Verification items for the finished model (mm, model axes). Give positions to 0.01 mm unless a question says otherwise; leave off trailing zeros. Write each loop counter-clockwise with the first axis right and the second up, starting at its lowest first coordinate (ties: lowest second). Pieces come first, ordered by that corner, then holes.
from build123d import *

# Parameters (mm, degrees)
F0_W     = 555
F0_H     = 70
F1_DEPTH = 45
F2_R     = 11.85
F3_DEPTH = 45.001
F4_R     = 12
F5_DEPTH = 45.001


with BuildPart() as f1:
    # F0 (on Front) → F1 (new body)
    with BuildSketch(Plane.XZ):
        with Locations((-277.5, -35)):
            Rectangle(F0_W, F0_H)
    extrude(amount=F1_DEPTH)

    # F2 (on face) → F3 (cut, through all)
    with BuildSketch(Plane(origin=(0, 0, 0), x_dir=(-1, 0, 0), z_dir=(0, 1, 0))):
        with Locations((525, -24)):
            Circle(F2_R)
    extrude(amount=-F3_DEPTH, mode=Mode.SUBTRACT)

    # F4 (on face) → F5 (cut, through all)
    with BuildSketch(Plane(origin=(0, 0, 0), x_dir=(-1, 0, 0), z_dir=(0, 1, 0))):
        with Locations((47, -24)):
            Circle(F4_R)
    extrude(amount=-F5_DEPTH, mode=Mode.SUBTRACT)


solid = f1.part
Item 1: Sectioned sample at A-A on z = -24. Record the cut outline in (x, y), then the cut area to 3 significant figures.
Answer key:
outline: (-555, -45) - (-536.85, -45) - (-536.85, 0) - (-555, 0) - close; (-513.15, -45) - (-59, -45) - (-59, 0) - (-513.15, 0) - close; (-35, -45) - (0, -45) - (0, 0) - (-35, 0) - close
area: 22,800 mm2
Item 2: Depth check by flat-ended pin: pin 1 (4 mm diameter, centred on y = -6.5, z = -39, fed in from +X). Enter the tip coordinate at first touch or a pass-through.
Answer key:
pin 1: stops at x = 0
Item 3: Sectioned sample at B-B on x = -47. Record the cut outline in (y, z), then the cut area to 3 significant figures.
Answer key:
outline: (-45, -70) - (0, -70) - (0, -36) - (-45, -36) - close; (-45, -12) - (0, -12) - (0, 0) - (-45, 0) - close
area: 2,070 mm2
Item 4: Sectioned sample at D-D on x = -525. Record the cut outline in (y, z), then the cut area to 3 significant figures.
Answer key:
outline: (-45, -70) - (0, -70) - (0, -35.85) - (-45, -35.85) - close; (-45, -12.15) - (0, -12.15) - (0, 0) - (-45, 0) - close
area: 2,080 mm2
Item 5: Sectioned sample at C-C on y = -23. Record the cut outline in (x, z).
Answer key:
outline: (-555, -70) - (0, -70) - (0, 0) - (-555, 0) - close; hole circle Ø23.7 at (-525, -24); hole circle Ø24 at (-47, -24)
Item 6: Release check for a two-part mould opening along Z. For faces 1 (the face through (-281, -45, -35)), 2 (the face through (-281, -22, 0)), 3 (the face through (-38.156, -22.185, -15.89)), 4 (the face through (-535.946, -22.185, -28.539)) record: released by +Z, released by -Z, zero draft, split by the parting line, or undercut.
Answer key:
face 1: zero draft
face 2: released by +Z
face 3: undercut
face 4: undercut
Item 7: Scan lines: line 1 along Z through (x, y) = (-525, -8.5); line 2 along Z through (x, y) = (-47, -9.5); line 3 along X through (y, z) = (-40, -32). Record each from-to range of solid material in increasing order.
Answer key:
line 1: z = -70 to -35.85, -12.15 to 0
line 2: z = -70 to -36, -12 to 0
line 3: x = -555 to -533.74, -516.26 to -55.94, -38.06 to 0
